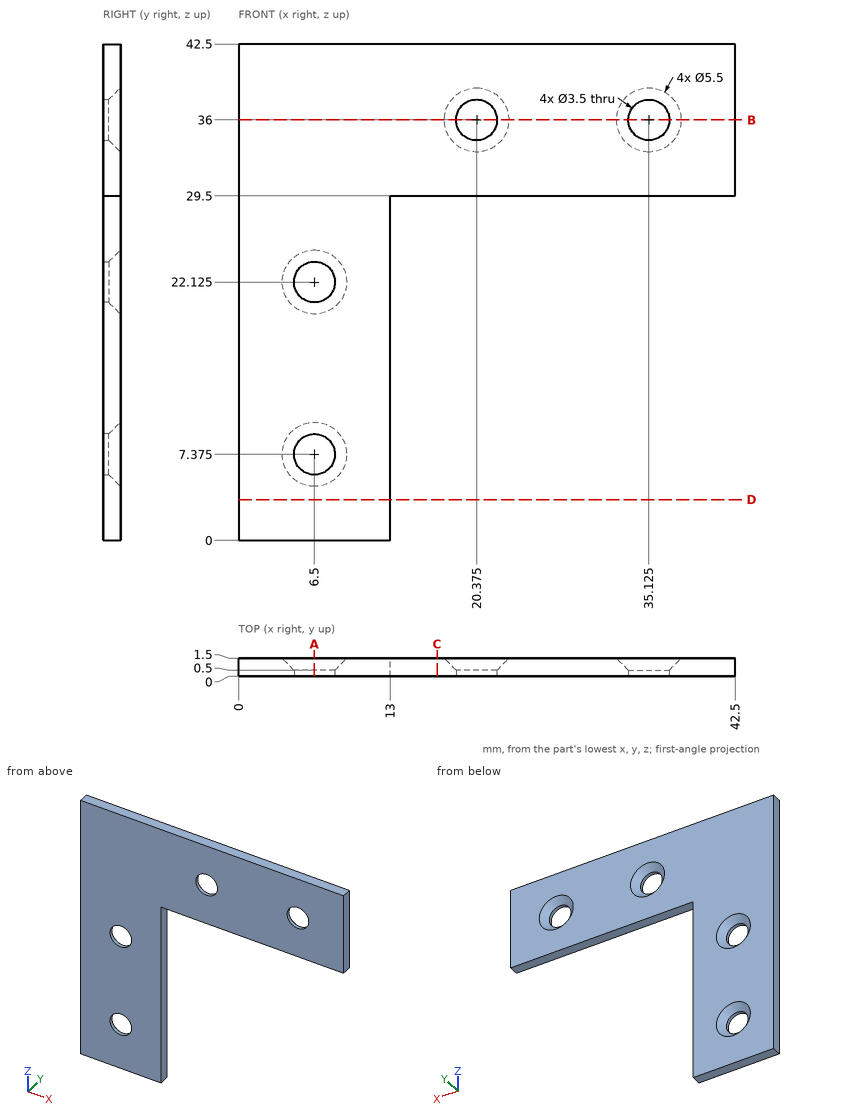
The drawing under review shows one solid part. Ordinate dimensions are in mm from its lowest x, y, z. Give positions to 0.01 mm unless a question says otherwise; leave off trailing zeros. Order: outer loops, then holes, each group sorted by start corner. A loop starts at its lowest first (then second) coordinate and runs counter-clockwise, first axis right, second up. Notation, with made-up numbers: M 34,-2.5 L 46,-2.5 A23 ccw 46,5.5 Z; hole C 80,-26.75 d5. An arc over 180 degrees is marked long. One line per question, with ' | ' between items. Start each with the question number.
Q1. For pin 1 Ø4 at (x, z) = (6.5, 7.375) entering from +Y; pin 2 Ø2 at (x, z) = (35.125, 36) entering from -Y, all flat-tipped, find the tip position at first contact; note any pin that passes through.
Q2. We need section B-B (z = 36). Write out the cut boundary in (x, y) (3 decimals), plus the area to 4 significant figures.
Q3. We need section C-C (x = 17). Write out the cut boundary in (y, z), plus the area to 3 significant figures.
Q4. For L1, parallel to X at y = 0.35, z = 36 (3 decimals); L2, parallel to X at y = 1.25, z = 34 (3 decimals); L3, parallel to Z at x = 8.5, y = 1.15, list the stretches that pass through material, from the lowest coordinate up. Write a range as [from, to].
Q5. We need section D-D (z = 3.5). Write out the cut boundary in (x, y).
Q6. We need section A-A (x = 6.5). Write out the cut boundary in (y, z) (3 decimals), plus the area to 4 significant figures.
Returned:
1) pin 1: y = 0.75 | pin 2: through
2) outline: M 0,0 L 18.625,0 L 18.625,0.5 L 17.625,1.5 L 0,1.5 Z; M 22.125,0 L 33.375,0 L 33.375,0.5 L 32.375,1.5 L 23.125,1.5 L 22.125,0.5 Z; M 36.875,0 L 42.5,0 L 42.5,1.5 L 37.875,1.5 L 36.875,0.5 Z | area: 51.25 mm2
3) outline: M 0,29.5 L 1.5,29.5 L 1.5,42.5 L 0,42.5 Z | area: 19.5 mm2
4) L1: [0, 18.625], [22.125, 33.375], [36.875, 42.5] | L2: [0, 18.875], [21.875, 33.625], [36.625, 42.5] | L3: [0, 6.05], [8.7, 20.8], [23.45, 42.5]
5) outline: M 0,0 L 13,0 L 13,1.5 L 0,1.5 Z
6) outline: M 0,0 L 1.5,0 L 1.5,4.625 L 0.5,5.625 L 0,5.625 Z; M 0,9.125 L 0.5,9.125 L 1.5,10.125 L 1.5,19.375 L 0.5,20.375 L 0,20.375 Z; M 0,23.875 L 0.5,23.875 L 1.5,24.875 L 1.5,42.5 L 0,42.5 Z | area: 51.25 mm2
